Build history of the part. All positions in model axes, mm. Face numbers are marked on the shaded views. A direction names the side the tool comes from. Round coordinates to 2 decimals unless told otherwise and drop trailing zeros. Loops run counter-clockwise (first coordinate to the right, second up) from the corner with the lowest first, then second, coordinate; pieces in that order, holes last. Notation, with made-up numbers: (21.5, -20) - (55.5, -20) arc R10 ccw to (55.5, -15) - close; hole circle Ø2 at (-32.5, 58). An arc over 180 degrees is marked (long way). Use one line per item in the form item = value. Start each with the question number.
Q1. Drill centre lines: line 1 (Z direction, x = 106, y = -6.75); line 2 (Z direction, x = 216, y = 5.75); line 3 (Z direction, x = 210.5, y = -7.75). Where is each one in solid material? Low to high.
Q2. Saw through at C-C (x = 74). Give the cut face in (y, z).
Q3. 3-axis set-ups, long thin cutter, end or side, ignore diameter. For the marked faces 1, 2 and 3: which of +Z, -Z, +X, -X, +Y, -Y reach the whole face in a straight line?
Q4. Pin check, flat tips, straight feed: pin 1 (2 mm diameter, centred on x = 208, z = 6.5, fed in from +Y); pin 2 (3.5 mm diameter, centred on y = -6.5, z = 8, fed in from -X); pin 3 (10 mm diameter, centred on x = 43.5, y = -4.5, fed in from -Z); pin 4 (5 mm diameter, centred on x = 111.5, y = -5, fed in from -Z). Stop position of each tip, or through.
Q5. Saw through at A-A (x = 155.5). Give the cut face in (y, z), then the cut area to 3 significant figures.
Q6. Mould opens along X. For the marked faces 4, 5 and 6 say: released by +X, released by -X, zero draft, split by the parting line, or undercut.
Q7. Saw through at D-D (x = 222.5). Give the cut face in (y, z), then the cut area to 3 significant figures.
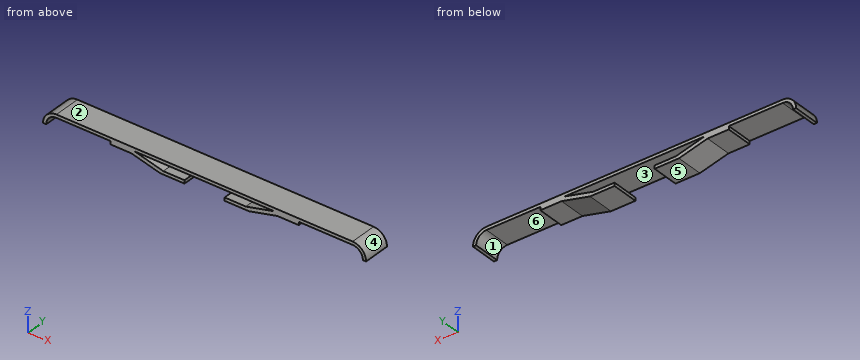
```python
from build123d import *

# Parameters (mm, degrees)
SKETCH1_W           = 304.8
SKETCH1_H           = 25.4
BOSS_EXTRUDE2_DEPTH = 12.7
FILLET1_R           = 12.7
CUT_EXTRUDE3_DEPTH  = 281.209703849
SKETCH8_W           = 70
SKETCH8_H           = 25.4
BOSS_EXTRUDE3_DEPTH = 9.7
CUT_EXTRUDE4_DEPTH  = 281.209703849
CUT_EXTRUDE5_DEPTH  = 281.209703849


with BuildPart() as part:
    # Sketch1 → Boss-Extrude2 (new body)
    with BuildSketch(Plane.XY):
        with Locations((126.366978193, -2.136448598)):
            Rectangle(SKETCH1_W, SKETCH1_H)
    extrude(amount=BOSS_EXTRUDE2_DEPTH)

    # Fillet1
    fillet1_edges = [part.edges().sort_by_distance(p)[0] for p in [
        (-26.033021807, -2.136448598, 12.7),
        (278.766978193, -2.136448598, 12.7),
    ]]
    fillet(fillet1_edges, radius=FILLET1_R - 0.0001)  # a hair under: the kernel refuses the full size

    # Sketch6 → Cut-Extrude3 (cut, through all)
    with BuildSketch(Plane(origin=(0, 10.563551402, 0), x_dir=(1, 0, 0), z_dir=(0, 1, 0))):
        with BuildLine():
            Line((-23.033021807, 0), (275.766978193, 0))
            ThreePointArc((275.766978193, 0), (272.925913971, -6.858935778), (266.066978193, -9.7))
            Line((266.066978193, -9.7), (-13.333021807, -9.7))
            ThreePointArc((-13.333021807, -9.7), (-20.191957584, -6.858935778), (-23.033021807, 0))
        make_face()
    extrude(amount=-CUT_EXTRUDE3_DEPTH, mode=Mode.SUBTRACT)

    # Sketch8 → Boss-Extrude3 (add)
    with BuildSketch(Plane(origin=(0, 0, 9.7), x_dir=(-1, 0, 0), z_dir=(0, 0, -1))):
        with Locations((-180.266978193, -2.136448598)):
            Rectangle(SKETCH8_W, SKETCH8_H)
        with Locations((-72.466978193, -2.136448598)):
            Rectangle(SKETCH8_W, SKETCH8_H)
    extrude(amount=BOSS_EXTRUDE3_DEPTH)

    # Sketch9 → Cut-Extrude4 (cut, through all)
    with BuildSketch(Plane(origin=(0, 10.563551402, 0), x_dir=(1, 0, 0), z_dir=(0, 1, 0))):
        Polygon((145.266978193, -9.7), (165.266978193, -9.7), (192.266978193, -9.7), (165.266978193, -3), (145.266978193, -3), align=None)
        Polygon((215.266978193, -6.7), (195.266978193, -6.7), (168.266978193, 0), (215.266978193, 0), align=None)
    extrude(amount=-CUT_EXTRUDE4_DEPTH, mode=Mode.SUBTRACT)

    # Sketch12 → Cut-Extrude5 (cut, through all)
    with BuildSketch(Plane(origin=(0, 10.563551402, 0), x_dir=(1, 0, 0), z_dir=(0, 1, 0))):
        Polygon((107.466978193, -9.7), (107.466978193, -3), (87.466978193, -3), (60.466978193, -9.7), align=None)
        Polygon((37.466978193, -6.7), (57.466978193, -6.7), (84.466978193, 0), (37.466978193, 0), align=None)
    extrude(amount=-CUT_EXTRUDE5_DEPTH, mode=Mode.SUBTRACT)


solid = part.part
```
Report:
q1.line_1 = 0 to 3, 9.7 to 12.7
q1.line_2 = 9.7 to 12.7
q1.line_3 = 6.7 to 12.7
q2.outline = (-14.84, 2.6) - (10.56, 2.6) - (10.56, 6.34) - (-14.84, 6.34) - close; (-14.84, 9.7) - (10.56, 9.7) - (10.56, 12.7) - (-14.84, 12.7) - close
q3.face_1 = -Z, +Y, -Y
q3.face_2 = +Z, +X, -X, +Y, -Y
q3.face_3 = +Y, -Y
q4.pin_1 = 10.56
q4.pin_2 = -24.39
q4.pin_3 = 6.7
q4.pin_4 = 9.7
q5.outline = (-14.84, 0) - (10.56, 0) - (10.56, 3) - (-14.84, 3) - close; (-14.84, 9.7) - (10.56, 9.7) - (10.56, 12.7) - (-14.84, 12.7) - close
q5.area = 152 mm²
q6.face_4 = released by +X
q6.face_5 = zero draft
q6.face_6 = undercut
q7.outline = (-14.84, 9.7) - (10.56, 9.7) - (10.56, 12.7) - (-14.84, 12.7) - close
q7.area = 76.2 mm²
